Geometry: final body of the model. Coordinates: model frame, mm. A direction names the side the tool comes from. Coordinates: 2 decimals unless noted, no trailing zeros. Loops run counter-clockwise (first coordinate to the right, second up) from the corner with the lowest first, then second, coordinate; pieces in that order, holes last. Notation, with made-up numbers: (0.25, 72.5) -> (24.25, 72.5) arc R30 cw to (24.25, 105.5) -> close; hole circle Ø2 at (18.25, 42.25). An arc over 180 degrees is marked (long way). One line per item, written item: value. Start each with the question number.
from build123d import *

# Parameters (mm, degrees)
SKETCH1_W           = 112.776
SKETCH1_H           = 96.774
BOSS_EXTRUDE1_DEPTH = 25.4
SKETCH2_R           = 8.334375
CUT_EXTRUDE2_DEPTH  = 151.760715215
SKETCH3_R           = 11.509375
CUT_EXTRUDE3_DEPTH  = 12.7
SKETCH4_R           = 11.509375
CUT_EXTRUDE4_DEPTH  = 12.7
SKETCH5_R           = 16.6497
CUT_EXTRUDE5_DEPTH  = 2.8194
SKETCH6_R           = 3.571875
CUT_EXTRUDE6_DEPTH  = 7.874
SKETCH8_R           = 3.175
CUT_EXTRUDE9_DEPTH  = 7.874
SKETCH9_R           = 3.175
BOSS_EXTRUDE2_DEPTH = 12.7


with BuildPart() as part:
    # Sketch1 → Boss-Extrude1 (new body)
    with BuildSketch(Plane.YZ):
        with Locations((56.388, 48.387)):
            Rectangle(SKETCH1_W, SKETCH1_H)
    extrude(amount=BOSS_EXTRUDE1_DEPTH)

    # Sketch2 → Cut-Extrude2 (cut, through all)
    with BuildSketch(Plane.YZ):
        with Locations(Location((15.875, 15.875, 0), (0, 0, 270))):
            Circle(SKETCH2_R)
        with Locations(Location((96.901, 15.875, 0), (0, 0, 270))):
            Circle(SKETCH2_R)
        with Locations(Location((15.875, 80.899, 0), (0, 0, 270))):
            Circle(SKETCH2_R)
        with Locations(Location((96.901, 80.899, 0), (0, 0, 270))):
            Circle(SKETCH2_R)
    extrude(amount=CUT_EXTRUDE2_DEPTH, mode=Mode.SUBTRACT)

    # Sketch3 → Cut-Extrude3 (cut)
    with BuildSketch(Plane.YZ):
        with Locations(Location((28.575, 48.387, 0), (0, 0, 270))):
            Circle(SKETCH3_R)
        with Locations(Location((74.549, 48.387, 0), (0, 0, 270))):
            Circle(SKETCH3_R)
    extrude(amount=CUT_EXTRUDE3_DEPTH, mode=Mode.SUBTRACT)

    # Sketch4 → Cut-Extrude4 (cut)
    with BuildSketch(Plane.YZ):
        with Locations((38.227, 48.387)):
            Circle(SKETCH4_R)
        with Locations((84.201, 48.387)):
            Circle(SKETCH4_R)
    extrude(amount=CUT_EXTRUDE4_DEPTH, mode=Mode.SUBTRACT)

    # Sketch5 → Cut-Extrude5 (cut)
    with BuildSketch(Plane.YZ):
        with Locations((38.227, 48.387)):
            Circle(SKETCH5_R)
        with Locations((84.201, 48.387)):
            Circle(SKETCH5_R)
    extrude(amount=CUT_EXTRUDE5_DEPTH, mode=Mode.SUBTRACT)

    # Sketch6 → Cut-Extrude6 (cut)
    with BuildSketch(Plane.YZ):
        with Locations(Location((105.537, 48.387, 0), (0, 0, 270))):
            Circle(SKETCH6_R)
        with Locations(Location((56.515, 15.875, 0), (0, 0, 270))):
            Circle(SKETCH6_R)
    extrude(amount=CUT_EXTRUDE6_DEPTH, mode=Mode.SUBTRACT)

    # Sketch8 → Cut-Extrude9 (cut)
    with BuildSketch(Plane.YZ):
        with Locations(Location((7.239, 48.387, 0), (0, 0, 270))):
            Circle(SKETCH8_R)
        with Locations(Location((56.261, 80.899, 0), (0, 0, 270))):
            Circle(SKETCH8_R)
    extrude(amount=CUT_EXTRUDE9_DEPTH, mode=Mode.SUBTRACT)

    # Sketch9 → Boss-Extrude2 (add)
    with BuildSketch(Plane.YZ):
        with Locations((0, 56.388)):
            Circle(SKETCH9_R)
    extrude(amount=BOSS_EXTRUDE2_DEPTH)


solid = part.part
1. Section C-C on y = 28.5. Return the cut outline in (x, z), plus the area to 3 significant figures.
2. Pin query (flat end, axial travel): pin 1 Ø1.5 at (x, y) = (12, 51.5) entering from -Z; pin 2 Ø8.5 at (y, z) = (44.5, 50.5) entering from -X; pin 3 Ø1.6 at (y, z) = (-1, 55) entering from +X; pin 4 Ø4 at (y, z) = (56.261, 80.899) entering from -X. Return the tip coordinate at first contact, or that it passes through.
3. Section B-B on x = 21. Return the cut outline in (y, z) (3 decimals), plus the area to 3 significant figures.
4. Set-up query: faces 1 (the face through (12.7, -1, 56)), 2 (the face through (12.52, 16.24, 24.2)), 3 (the face through (2.819, 50, 46)). Return all of +Z, -Z, +X, -X, +Y, -Y with unobstructed straight access to the full face (end or side cutting, diameter ignored); none if empty.
5. Section D-D on x = 6.5. Count the separate pieces of the cut face and the enclosed holes in it, plus the area to 3 significant figures.
6. Line query: L1, parallel to Y at x = 3.75, z = 77; L2, parallel to Y at x = 9.75, z = 50.5; L3, parallel to Z at x = 13, y = 18. Output: solid intervals per line, ascending. Write a range as [from, to].
7. Section A-A on z = 79. Return the cut outline in (x, y).
8. Draft query along Z for faces 4 (the face through (0, 54, 60)), 5 (the face through (6.261, -3.174, 56.458)), 6 (the face through (12.7, 34, 49)). Return one class per face: released by +Z, released by -Z, zero draft, split by the parting line, or undercut.
Checks:
1. outline: (0, 0) -> (25.4, 0) -> (25.4, 96.77) -> (0, 96.77) -> (0, 61.9) -> (2.82, 61.9) -> (2.82, 59.9) -> (12.7, 59.9) -> (12.7, 36.88) -> (2.82, 36.88) -> (2.82, 34.87) -> (0, 34.87) -> close
1. area: 2,150 mm²
2. pin 1: z = 0
2. pin 2: x = 12.7
2. pin 3: x = 12.7
2. pin 4: x = 7.87
3. outline: (0, 0) -> (112.776, 0) -> (112.776, 96.774) -> (0, 96.774) -> close; hole circle Ø16.669 at (15.875, 15.875); hole circle Ø16.669 at (15.875, 80.899); hole circle Ø16.669 at (96.901, 15.875); hole circle Ø16.669 at (96.901, 80.899)
3. area: 10,000 mm²
4. face 1: +Z, -Z, +X, -Y
4. face 2: +X, -X
4. face 3: -X
5. separate pieces: 1
5. enclosed holes: 10
5. area: 8,650 mm²
6. L1: [0, 8.51], [23.24, 89.53], [104.27, 112.78]
6. L2: [0, 17.26], [49.54, 63.24], [95.51, 112.78]
6. L3: [0, 7.82], [23.93, 72.84], [88.96, 96.77]
7. outline: (0, 0) -> (25.4, 0) -> (25.4, 7.76) -> (0, 7.76) -> close; (0, 23.99) -> (25.4, 23.99) -> (25.4, 88.79) -> (0, 88.79) -> (0, 58.81) -> (7.87, 58.81) -> (7.87, 53.72) -> (0, 53.72) -> close; (0, 105.02) -> (25.4, 105.02) -> (25.4, 112.78) -> (0, 112.78) -> close
8. face 4: zero draft
8. face 5: split by the parting line
8. face 6: undercut
